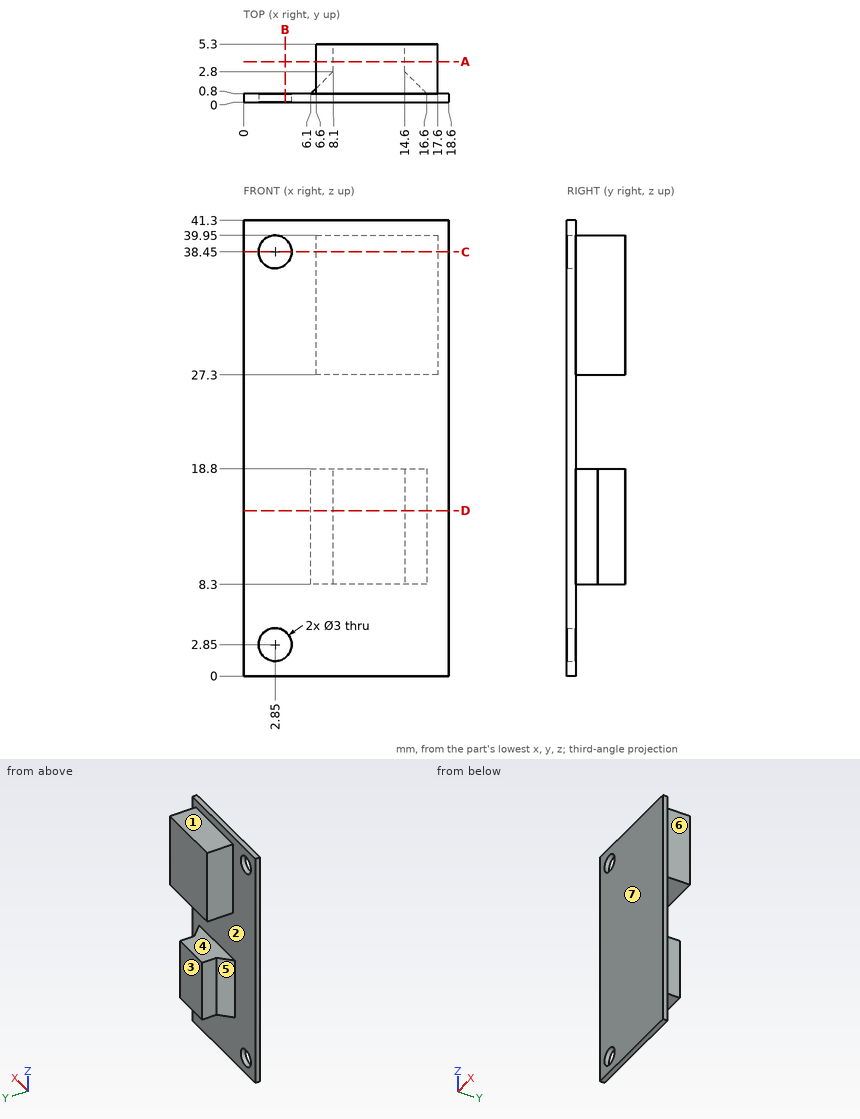
Can you work these out from the drawing? Everything is in mm from the part's minimum corner. A direction names the side the tool comes from. Round coordinates to 2 decimals unless told otherwise and drop trailing zeros. Loops run counter-clockwise (first coordinate to the right, second up) from the corner with the lowest first, then second, coordinate; pieces in that order, holes last. Notation, with made-up numbers: (-24, 34) -> (32, 34) arc R25 ccw to (32, 70) -> close; hole circle Ø6 at (-17, 58.5). An arc over 180 degrees is marked (long way). Answer in a Markdown table with one row per item.
Item 1: If I drill on probe 1 along Z at (x, y) = (2.85, 0.3); probe 2 along X at (y, z) = (0.5, 2.85); probe 3 along Z at (x, y) = (13, 0.85), over which ranges is the centre line in solid material (lowest first)?
Answer block:
| item | result |
|---|---|
| probe 1 | 0 to 1.35, 4.35 to 36.95, 39.95 to 41.3 |
| probe 2 | 0 to 1.35, 4.35 to 18.6 |
| probe 3 | 8.3 to 18.8, 27.3 to 39.95 |
Item 2: Suppose I cut it at D-D, the plane z = 15. List the corners of the cut face in (x, y) for me, plus the area to 3 significant figures.
Answer block:
| item | result |
|---|---|
| outline | (0, 0) -> (18.6, 0) -> (18.6, 0.8) -> (16.6, 0.8) -> (14.6, 2.8) -> (14.6, 5.3) -> (8.1, 5.3) -> (8.1, 2.8) -> (6.1, 0.8) -> (0, 0.8) -> close |
| area | 48.1 mm² |
Item 3: Suppose I cut it at B-B, the plane x = 3.75. List the corners of the cut face in (y, z) for me, plus the area to 3 significant figures.
Answer block:
| item | result |
|---|---|
| outline | (0, 0) -> (0.8, 0) -> (0.8, 1.65) -> (0, 1.65) -> close; (0, 4.05) -> (0.8, 4.05) -> (0.8, 37.25) -> (0, 37.25) -> close; (0, 39.65) -> (0.8, 39.65) -> (0.8, 41.3) -> (0, 41.3) -> close |
| area | 29.2 mm² |
Item 4: We'd pull the mould along Z, two halves only. Please class the marked faces 1, 2 and 3: released by +Z, released by -Z, zero draft, split by the parting line, or undercut.
Answer block:
| item | result |
|---|---|
| face 1 | released by +Z |
| face 2 | undercut |
| face 3 | zero draft |
Item 5: Suppose I cut it at A-A, the plane y = 3.7. List the corners of the cut face in (x, z) for me, plus the area to 3 significant figures.
Answer block:
| item | result |
|---|---|
| outline | (6.6, 27.3) -> (17.6, 27.3) -> (17.6, 39.95) -> (6.6, 39.95) -> close; (8.1, 8.3) -> (14.6, 8.3) -> (14.6, 18.8) -> (8.1, 18.8) -> close |
| area | 207 mm² |
Item 6: Suppose I cut it at C-C, the plane z = 38.45. List the corners of the cut face in (x, y) for me, plus the area to 3 significant figures.
Answer block:
| item | result |
|---|---|
| outline | (0, 0) -> (1.35, 0) -> (1.35, 0.8) -> (0, 0.8) -> close; (4.35, 0) -> (18.6, 0) -> (18.6, 0.8) -> (17.6, 0.8) -> (17.6, 5.3) -> (6.6, 5.3) -> (6.6, 0.8) -> (4.35, 0.8) -> close |
| area | 62.0 mm² |
Item 7: Will these pins go through, and if not, where does the flat tip stop? P1, Ø1.3, axis at x = 13.5, y = 2.5, coming from the +Z side; P2, Ø1.3, axis at y = 3.5, z = 34, coming from the -X side; P3, Ø4, axis at x = 5, z = 24.5, coming from the +Y side.
Answer block:
| item | result |
|---|---|
| P1 | z = 39.95 |
| P2 | x = 6.6 |
| P3 | y = 0.8 |
Item 8: On a 3-axis mill with a long thin cutter (end or side, diameter ignored), from which of +Z, -Z, +X, -X, +Y, -Y can I reach the whole of each face in a straight line? I mean the marked faces 4, 5, 6 and 7. Say none if no direction works.
Answer block:
| item | result |
|---|---|
| face 4 | +X, -X, +Y |
| face 5 | -Z, -X, +Y |
| face 6 | +Z, -Z, +X, +Y |
| face 7 | +Z, -Z, +X, -X, -Y |
